Could you check a few things on this drawing? It's one solid part, dimensions in mm from its lowest x, y, z. A direction names the side the tool comes from. Round coordinates to 2 decimals unless told otherwise and drop trailing zeros. Loops run counter-clockwise (first coordinate to the right, second up) from the corner with the lowest first, then second, coordinate; pieces in that order, holes last. Notation, with made-up numbers: M 65.25,52 L 80.25,52 A14 cw 80.25,67 Z; hole C 29.5,34 d7. An arc over 180 degrees is marked long. Put each result on its own line as item: value. Start each with the question number.
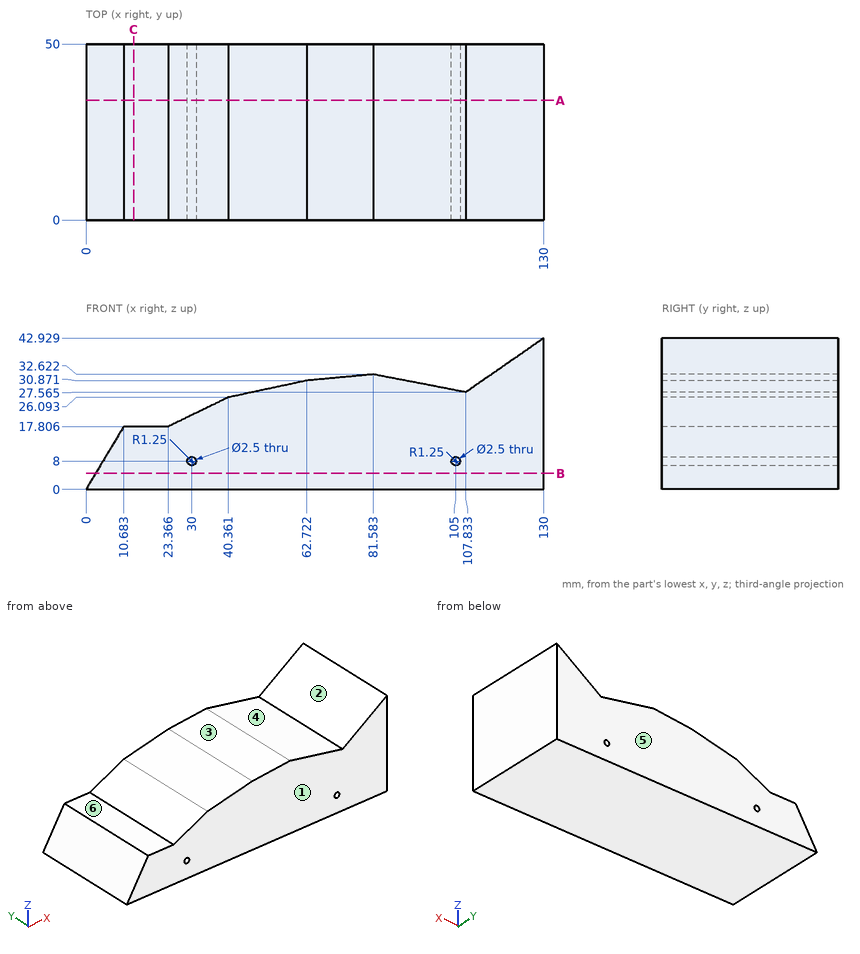
1) Suppose I cut it at C-C (x = 13.5). Write out the boundary of the cut face in (y, z) (1 decimal), plus the area to 3 significant figures.
2) If I drill on probe 1 along X at (y, z) = (28, 8); probe 2 along Z at (x, y) = (30, 12); probe 3 along Z at (x, y) = (105, 24), over which ranges is the centre line in solid material (lowest first)? Write a range as from..to.
3) I'm going to push flat-ended pins straight in: P1, Ø12, axis at x = 77, y = 38, coming from the +Z side; P2, Ø1, axis at x = 66, y = 39, coming from the +Z side; P3, Ø10, axis at y = 21.5, z = 18.5, coming from the -X side; P4, Ø2, axis at x = 30, z = 8, coming from the -Y side. Where does each tip first touch, or does it pass through?
4) If we mould it in two halves opening along X, with no side actions, what happens to the marked faces 1, 2 and 3? For each: pulls with the +X half, pulls with the -X half, needs draft (parallel to the pull), parting line crosses it, or undercut.
5) Suppose I cut it at B-B (z = 4.5). Write out the boundary of the cut face in (x, y), plus the area to 4 significant figures.
6) Suppose I cut it at A-A (y = 34). State how many separate pieces and enclosed holes the cut face has, plus the area to 3 significant figures.
7) On a 3-axis mill with a long thin cutter (end or side, diameter ignored), from which of +Z, -Z, +X, -X, +Y, -Y can I reach the whole of each face in a straight line? I mean the marked faces 4, 5 and 6. Say none if no direction works.
Results are:
1. outline: M 0,0 L 50,0 L 50,17.8 L 0,17.8 Z
1. area: 890 mm²
2. probe 1: 4.8..28.75, 31.25..103.75, 106.25..130
2. probe 2: 0..6.75, 9.25..21.04
2. probe 3: 0..6.75, 9.25..28.11
3. P1: z = 32.62
3. P2: z = 31.22
3. P3: x = 8.1
3. P4: through
4. face 1: needs draft
4. face 2: undercut
4. face 3: pulls with the -X half
5. outline: M 2.7,0 L 130,0 L 130,50 L 2.7,50 Z
5. area: 6,365 mm²
6. separate pieces: 1
6. enclosed holes: 2
6. area: 3,490 mm²
7. face 4: +Z, +Y, -Y
7. face 5: +Z, -Z, +X, -X, +Y
7. face 6: +Z, -X, +Y, -Y
